from build123d import *

# Parameters (mm, degrees)
SKETCH_1_W               = 50
SKETCH_1_H               = 50
EXTRUDE_1_DEPTH          = 30
SKETCH_2_W               = 58
SKETCH_2_H               = 58
EXTRUDE_2_DEPTH          = 8.75
SKETCH_3_W               = 58
SKETCH_3_H               = 58
EXTRUDE_3_DEPTH          = 8.75
SKETCH_6_R               = 4
EXTRUDE_4_DEPTH          = 18.25
SKETCH_4_OUTSIDE_W       = 81.024
SKETCH_4_OUTSIDE_H       = 81.024
SKETCH_4_OUTSIDE_R       = 34
CUT_EXTRUDE_2_DEPTH      = 63.755477849
HOLE_WIZARD_M3_5_1_D     = 2.9
HOLE_WIZARD_M3_5_1_DEPTH = 8
HOLE_WIZARD_M3_5_1_TIP   = 0.871247898


with BuildPart() as part:
    # 草图1 → 凸台-拉伸1 (new body)
    with BuildSketch(Plane.XY):
        Rectangle(SKETCH_1_W, SKETCH_1_H)
    extrude(amount=EXTRUDE_1_DEPTH)

    # 草图2 → 凸台-拉伸2 (add)
    with BuildSketch(Plane.XY.offset(30)):
        Rectangle(SKETCH_2_W, SKETCH_2_H)
    extrude(amount=EXTRUDE_2_DEPTH)

    # 草图3 → 凸台-拉伸3 (add)
    with BuildSketch(Plane(origin=(0, 0, 0), x_dir=(-1, 0, 0), z_dir=(0, 0, -1))):
        Rectangle(SKETCH_3_W, SKETCH_3_H)
    extrude(amount=EXTRUDE_3_DEPTH)

    # 草图6 → 凸台-拉伸4 (add)
    with BuildSketch(Plane.XY.offset(38.75)):
        Circle(SKETCH_6_R)
    extrude(amount=EXTRUDE_4_DEPTH)

    # 草图4 outside → 切除-拉伸2 (cut, through all)
    with BuildSketch(Plane.XY.offset(38.75)):
        Rectangle(SKETCH_4_OUTSIDE_W, SKETCH_4_OUTSIDE_H)
        Circle(SKETCH_4_OUTSIDE_R, mode=Mode.SUBTRACT)
    extrude(amount=-CUT_EXTRUDE_2_DEPTH, mode=Mode.SUBTRACT)

    # M3.5 螺纹孔1
    with Locations(Plane.XY.offset(38.75)):
        with Locations((0, 22.35), (-21.92, 0.43), (21.92, 0.43)):
            Hole(HOLE_WIZARD_M3_5_1_D / 2, depth=HOLE_WIZARD_M3_5_1_DEPTH)
            with Locations((0, 0, -(HOLE_WIZARD_M3_5_1_DEPTH + HOLE_WIZARD_M3_5_1_TIP / 2))):  # 118° drill point
                Cone(0, HOLE_WIZARD_M3_5_1_D / 2, HOLE_WIZARD_M3_5_1_TIP, mode=Mode.SUBTRACT)


solid = part.part
Model file for the job. Use its own axes, mm. A direction names the side the tool comes from. Give positions to 0.01 mm unless a question says otherwise; leave off trailing zeros. Write each loop counter-clockwise with the first axis right and the second up, starting at its lowest first coordinate (ties: lowest second). Pieces come first, ordered by that corner, then holes. Notation, with made-up numbers: M 56.25,54.25 L 83.25,54.25 A14 cw 83.25,77.25 Z; hole C 59.5,69 d2. An arc over 180 degrees is marked long. One line per item, written item: value. Start each with the question number.
Q1. 3-axis set-ups, long thin cutter, end or side, ignore diameter. For faces 4 (the flat face through (0, -25, 15)), 5 (the flat face through (-27, 0, 30)), 6 (the cylindrical face through (-22.589, -0.856, 34.694)): which of +Z, -Z, +X, -X, +Y, -Y reach the whole face in a straight line?
Q2. Probe probe 1 along X at (y, z) = (0.43, 35.25); probe 2 along Y at (x, z) = (0, 34); probe 3 along X at (y, z) = (0, 33). List the from-to ranges inside material, lowest first. Write a range as [from, to].
Q3. Two-plate mould, pull along Z, no slides. Class faces 1 (the flat face through (0, 29, 34)), 2 (the flat face through (0, 0, 57)), 3 (the flat face through (0, 27, 30)): +Z half, -Z half, draft (parallel to the pull), parting line (faces both ways), or undercut.
Q4. Drop flat-ended pins along their axis: pin 1 Ø4.5 at (x, y) = (26.5, -9) entering from +Z; pin 2 Ø1.5 at (y, z) = (-20.5, 35) entering from +X; pin 3 Ø9 at (y, z) = (-1, 8.5) entering from +X; pin 4 Ø12 at (x, z) = (11.5, 50) entering from -Y (3 decimals). Give the stop position or say it passes through.
Q5. Saw through at A-A, the plane y = 15. Write the cut outline in (x, z).
Q6. Saw through at B-B, the plane z = 18. Write the cut outline in (x, y), plus the area to 3 significant figures.
Output values:
1. face 4: +X, -X, -Y
1. face 5: -X, +Y, -Y
1. face 6: +Z
2. probe 1: x = [-29, -23.37], [-20.47, 20.47], [23.37, 29]
2. probe 2: y = [-29, 20.9], [23.8, 29]
2. probe 3: x = [-29, -23.3], [-20.54, 20.54], [23.3, 29]
3. face 1: draft
3. face 2: +Z half
3. face 3: undercut
4. pin 1: stops at z = 38.75
4. pin 2: stops at x = 27.68
4. pin 3: stops at x = 25
4. pin 4: passes through
5. outline: M -29,-8.75 L 29,-8.75 L 29,0 L 25,0 L 25,30 L 29,30 L 29,38.75 L -29,38.75 L -29,30 L -25,30 L -25,0 L -29,0 Z
6. outline: M -25,-23.04 A34 ccw -23.04,-25 L 23.04,-25 A34 ccw 25,-23.04 L 25,23.04 A34 ccw 23.04,25 L -23.04,25 A34 ccw -25,23.04 Z
6. area: 2,490 mm²
